from build123d import *

# Parameters (mm, degrees)
SZKIC4_R                   = 6
WYTNIJ_WYCI_GNI_CIE1_DEPTH = 10
SZKIC5_R                   = 6
WYTNIJ_WYCI_GNI_CIE2_DEPTH = 10
SZKIC6_R                   = 35
WYTNIJ_WYCI_GNI_CIE3_DEPTH = 15
WYTNIJ_WYCI_GNI_CIE4_START = -5
SZKIC7_R                   = 45
SZKIC7_R_2                 = 35
WYTNIJ_WYCI_GNI_CIE4_DEPTH = 5
SZKIC8_R                   = 25
WYTNIJ_WYCI_GNI_CIE5_DEPTH = 70
ZAOKR_GLENIE1_R            = 4
SZKIC9_W                   = 2
SZKIC9_H                   = 3


with BuildPart() as part:
    # Szkic2 → Obrót1 (revolve)
    with BuildSketch(Plane.XY, mode=Mode.PRIVATE) as obr_t1_sk:
        Polygon((82, 0), (82, 45), (66, 45), (66, 69.5), (56, 69.5), (56, 45), (25, 45), (25, 69.5), (15, 69.5), (15, 39.5), (0, 39.5), (0, 0), align=None)
    revolve(obr_t1_sk.sketch.rotate(Axis((0, 0, 0), (1, 0, 0)), 90), axis=Axis((0, 0, 0), (1, 0, 0)))

    # Szkic4 → Wytnij-wyciągnięcie1 (cut)
    with BuildSketch(Plane(origin=(66, 0, 0), x_dir=(0, 0, -1), z_dir=(1, 0, 0))):
        with Locations((0, 55)):
            Circle(SZKIC4_R)
        with Locations((55, 0)):
            Circle(SZKIC4_R)
        with Locations((0, -55)):
            Circle(SZKIC4_R)
        with Locations((-55, 0)):
            Circle(SZKIC4_R)
    extrude(amount=-WYTNIJ_WYCI_GNI_CIE1_DEPTH, mode=Mode.SUBTRACT)

    # Szkic5 → Wytnij-wyciągnięcie2 (cut)
    with BuildSketch(Plane.ZY.offset(-15)):
        with Locations((0, 60)):
            Circle(SZKIC5_R)
        with Locations((57.063390978, 18.541019662)):
            Circle(SZKIC5_R)
        with Locations((35.267115138, -48.541019662)):
            Circle(SZKIC5_R)
        with Locations((-35.267115138, -48.541019662)):
            Circle(SZKIC5_R)
        with Locations((-57.063390978, 18.541019662)):
            Circle(SZKIC5_R)
    extrude(amount=-WYTNIJ_WYCI_GNI_CIE2_DEPTH, mode=Mode.SUBTRACT)

    # Szkic6 → Wytnij-wyciągnięcie3 (cut)
    with BuildSketch(Plane.ZY):
        Circle(SZKIC6_R)
    extrude(amount=-WYTNIJ_WYCI_GNI_CIE3_DEPTH, mode=Mode.SUBTRACT)

    # Szkic7 → Wytnij-wyciągnięcie4 (cut)
    with BuildSketch(Plane(origin=(82, 0, 0), x_dir=(0, 0, -1), z_dir=(1, 0, 0)).offset(WYTNIJ_WYCI_GNI_CIE4_START)):
        with Locations(Location((0, 0, 0), (0, 0, 180))):
            Circle(SZKIC7_R)
        with Locations(Location((0, 0, 0), (0, 0, 180))):
            Circle(SZKIC7_R_2, mode=Mode.SUBTRACT)
    extrude(amount=WYTNIJ_WYCI_GNI_CIE4_DEPTH, mode=Mode.SUBTRACT)

    # Szkic8 → Wytnij-wyciągnięcie5 (cut)
    with BuildSketch(Plane(origin=(82, 0, 0), x_dir=(0, 0, -1), z_dir=(1, 0, 0))):
        Circle(SZKIC8_R)
    extrude(amount=-WYTNIJ_WYCI_GNI_CIE5_DEPTH, mode=Mode.SUBTRACT)

    # Zaokrąglenie1
    zaokr_glenie1_edges = [part.edges().sort_by_distance(p)[0] for p in [
        (82, 0, -35),
        (82, 0, 25),
    ]]
    fillet(zaokr_glenie1_edges, radius=ZAOKR_GLENIE1_R)

    # Szkic9 → Wycięcie-obrót1 (revolve, cut)
    with BuildSketch(Plane.XY, mode=Mode.PRIVATE) as wyci_cie_obr_t1_sk:
        with Locations((28, 43.5)):
            Rectangle(SZKIC9_W, SZKIC9_H)
    revolve(wyci_cie_obr_t1_sk.sketch.rotate(Axis((-4.1, 0, 0), (1, 0, 0)), 90), axis=Axis((-4.1, 0, 0), (1, 0, 0)), mode=Mode.SUBTRACT)


solid = part.part
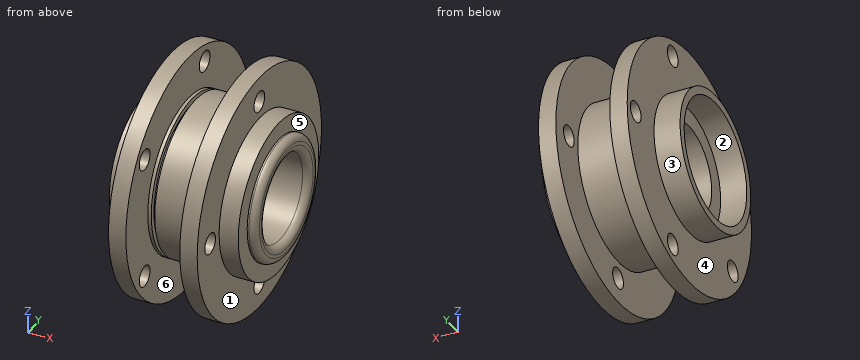
Build history of the part. All positions in model axes, mm. Face numbers are marked on the shaded views. A direction names the side the tool comes from. Coordinates: 2 decimals unless noted, no trailing zeros. Order: outer loops, then holes, each group sorted by start corner. A loop starts at its lowest first (then second) coordinate and runs counter-clockwise, first axis right, second up. Notation, with made-up numbers: (35.5, -25.5) - (59.5, -25.5) arc R20 cw to (59.5, -17.5) - close; hole circle Ø8 at (61, 3). An arc over 180 degrees is marked (long way). Put each result on its own line as item: value.
1. Saw through at B-B (x = 48). Write the cut outline in (y, z).
Answer sheet:
outline: circle Ø90 at (0, 0); hole circle Ø50 at (0, 0)
2. Tool access for the marked faces 4, 5 and 6: list every direction of +Z, -Z, +X, -X, +Y, -Y with a clear straight run to the whole face (end or side of a thin tool).
Answer sheet:
face 4: -X
face 5: +X
face 6: none
3. Saw through at C-C (z = 0). Give the number of separate pieces and of enclosed holes in the cut face, and give its area (3 significant figures).
Answer sheet:
separate pieces: 5
enclosed holes: 0
area: 3,310 mm^2
4. Pull direction Y, two halves, no side cores. Call the marked faces 1, 2 and 3: pulls with the +Y half, pulls with the -Y half, needs draft (parallel to the pull), parting line crosses it, or undercut.
Answer sheet:
face 1: needs draft
face 2: undercut
face 3: parting line crosses it
5. Probe line 1 along Y through (x, z) = (63, 0); line 2 along X through (y, z) = (33, -58); line 3 along Y through (x, z) = (9.5, -24.5) (3 decimals). List the from-to ranges inside material, lowest first. Write a range as [from, to].
Answer sheet:
line 1: y = [-69.5, -61], [-49, -25], [25, 49], [61, 69.5]
line 2: x = [15, 25], [56, 66]
line 3: y = [-30.984, -24.995], [24.995, 30.984]
6. Drop flat-ended pins along their axis: P1, Ø2, axis at x = 54.5, y = -35.5, coming from the +Z side; P2, Ø10, axis at x = 47, z = 6.5, coming from the -Y side (3 decimals); P3, Ø14, axis at y = -55, z = 0, coming from the -X side. Give the stop position or say it passes through.
Answer sheet:
P1: stops at z = 28.89
P2: stops at y = -44.975
P3: stops at x = 15
7. Saw through at D-D (x = 22.5). Write the cut outline in (y, z), and give its area (3 significant figures).
Answer sheet:
outline: circle Ø139 at (0, 0); hole circle Ø12 at (-48.54, -35.27); hole circle Ø12 at (-48.54, 35.27); hole circle Ø50 at (0, 0); hole circle Ø12 at (18.54, -57.06); hole circle Ø12 at (18.54, 57.06); hole circle Ø12 at (60, 0)
area: 12,600 mm^2
8. Saw through at A-A (z = 55). Write the cut outline in (x, y), and give its area (3 significant figures).
Answer sheet:
outline: (15, -42.49) - (25, -42.49) - (25, 12.91) - (15, 12.91) - close; (15, 24.18) - (25, 24.18) - (25, 42.49) - (15, 42.49) - close; (56, -42.49) - (66, -42.49) - (66, -6) - (56, -6) - close; (56, 6) - (66, 6) - (66, 42.49) - (56, 42.49) - close
area: 1,470 mm^2
